For this review, take the finished solid that the model builds, in its own axes (mm). Face numbers are marked on the shaded views. Coordinates: 2 decimals unless noted, no trailing zeros. Write each loop counter-clockwise with the first axis right and the second up, starting at its lowest first coordinate (ties: lowest second). Pieces come first, ordered by that corner, then holes. Notation, with made-up numbers: (-4.75, 40.5) -> (0.25, 40.5) arc R14 cw to (0.25, 49.5) -> close; hole circle Ø9 at (-14.75, -7.5). An arc over 180 degrees is marked (long way). One line per item, written item: value. Start each with the question number.
1) For probe 1 along Y at (x, z) = (5, 1.5); probe 2 along Y at (x, z) = (5, 2.3); probe 3 along Y at (x, z) = (14, 1.6), list the stretches that pass through material, from the lowest coordinate up. Write a range as from..to.
2) Add section A-A (y = -2). State the section outline as (x, z) points, and give its area (3 significant figures).
3) Mouldability with a two-part tool opening along Y and no side actions: class the marked faces 1, 2 and 3 as released by +Y, released by -Y, zero draft, split by the parting line, or undercut.
4) Add section D-D (x = 21.5). State the section outline as (y, z) points.
5) Add section B-B (z = 1.65). State the section outline as (x, y) points, and give its area (3 significant figures).
6) Add section C-C (x = -12). State the section outline as (y, z) points.
from build123d import *

# Parameters (mm, degrees)
CYLINDER001_R               = 4
CYLINDER001_DEPTH           = 4
CYLINDER001_PLACEMENT_ANGLE = 45
CYLINDER002_R               = 4
CYLINDER002_DEPTH           = 10
TORUS_R                     = 2
TORUS_ANGLE                 = 120
CYLINDER_R                  = 25
CYLINDER_DEPTH              = 3


with BuildPart() as cilindre001:
    # Cylinder001 → Cylinder001 (new body)
    with BuildSketch(Plane.XY):
        Circle(CYLINDER001_R)
    extrude(amount=CYLINDER001_DEPTH)


with BuildPart() as cilindre001_1:
    # Cylinder001 placement: moved
    add(cilindre001.part.moved(Location((5, -11, 1))).rotate(Axis((5, -11, 1), (0, 0, 1)), CYLINDER001_PLACEMENT_ANGLE))


with BuildPart() as cilindre002:
    # Cylinder002 → Cylinder002 (new body)
    with BuildSketch(Plane(origin=(-12, -2, 1), x_dir=(1, 0, 0), z_dir=(0, 0, 1))):
        Circle(CYLINDER002_R)
    extrude(amount=CYLINDER002_DEPTH)


with BuildPart() as torus:
    # Torus → Torus (revolve)
    with BuildSketch(Plane(origin=(0, 0, 2), x_dir=(1, 0, 0), z_dir=(0, -1, 0))):
        with Locations((15, 0)):
            Circle(TORUS_R)
    revolve(axis=Axis((0, 0, 2), (0, 0, 1)), revolution_arc=TORUS_ANGLE)


with BuildPart() as cut002:
    # Cylinder → Cylinder (new body)
    with BuildSketch(Plane.XY):
        Circle(CYLINDER_R)
    extrude(amount=CYLINDER_DEPTH)

    # Cut: cut Torus
    add(torus.part, mode=Mode.SUBTRACT)

    # Cut001: cut Cilindre002
    add(cilindre002.part, mode=Mode.SUBTRACT)

    # Cut002: cut Cilindre001
    add(cilindre001_1.part, mode=Mode.SUBTRACT)


solid = cut002.part
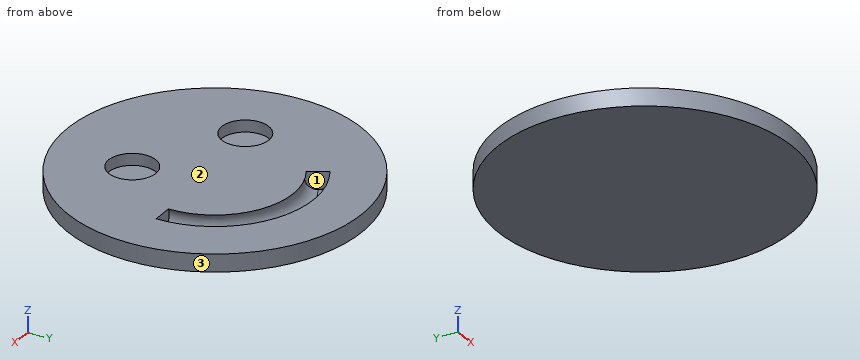
Numbers:
1. probe 1: -24.49..-15, -7..12.07, 16.18..24.49
1. probe 2: -24.49..-15, -7..12.02, 16.22..24.49
1. probe 3: -20.71..0, 9.57..20.71
2. outline: (-24.92, 0) -> (24.92, 0) -> (24.92, 3) -> (-8, 3) -> (-8, 1) -> (-16, 1) -> (-16, 3) -> (-24.92, 3) -> close
2. area: 134 mm²
3. face 1: undercut
3. face 2: zero draft
3. face 3: split by the parting line
4. outline: (-12.76, 0) -> (12.76, 0) -> (12.76, 3) -> (-12.76, 3) -> close
5. outline: circle Ø50 at (0, 0); hole circle Ø8 at (-12, -2); hole (-8.48, 14.7) -> (-6.52, 11.29) arc R13.03 cw to (13.03, 0) -> (16.97, 0) arc R16.97 ccw to start; hole circle Ø8 at (5, -11)
5. area: 1,740 mm²
6. outline: (-21.93, 0) -> (21.93, 0) -> (21.93, 3) -> (2, 3) -> (2, 1) -> (-6, 1) -> (-6, 3) -> (-21.93, 3) -> close
